from build123d import *

# Parameters (mm, degrees)
BOSS_EXTRUDE1_DEPTH     = 172
BOSS_EXTRUDE2_DEPTH     = 20
SKETCH2_W               = 10
SKETCH2_H               = 13
BOSS_EXTRUDE3_DEPTH     = 15
SKETCH6_W               = 7
SKETCH6_H               = 82.975623271
BOSS_EXTRUDE4_DEPTH     = 15
SKETCH9_W               = 249.172322426
SKETCH9_H               = 172
BOSS_EXTRUDE7_DEPTH     = 20
CUT_EXTRUDE3_DEPTH      = 75
CUT_EXTRUDE3_DEPTH_BACK = 75
SKETCH11_W              = 220
SKETCH11_H              = 130
CUT_EXTRUDE4_DEPTH      = 135
CUT_EXTRUDE4_DEPTH_BACK = 5
SKETCH12_W              = 220
SKETCH12_H              = 10
FILLET2_R               = 70


with BuildPart() as part:
    # Sketch1 → Boss-Extrude1 (new body)
    with BuildSketch(Plane(origin=(0, 0, 0), x_dir=(1, 0, 0), z_dir=(0, 1, 0))):
        Polygon((-125, -75), (-125, -85), (125, -85), (125, 85), (-125, 85), (-125, 75), (115, 75), (115, -75), align=None)
    extrude(amount=BOSS_EXTRUDE1_DEPTH)

    # Sketch1<3> → Boss-Extrude2 (add)
    with BuildSketch(Plane(origin=(0, 0, 0), x_dir=(1, 0, 0), z_dir=(0, 1, 0))):
        Polygon((-195, -85), (-125, -85), (-125, -75), (115, -75), (115, 75), (-125, 75), (-125, 105), (-195, 105), align=None)
    extrude(amount=BOSS_EXTRUDE2_DEPTH)

    # Sketch2 → Boss-Extrude3 (add)
    with BuildSketch(Plane.XY.offset(-75)):
        with Locations((-120, 155.5)):
            Rectangle(SKETCH2_W, SKETCH2_H)
    boss_extrude3 = extrude(amount=BOSS_EXTRUDE3_DEPTH)

    # Sketch5 → CBORE for M3 Hex Head Cap Screw1 (revolve, cut)
    with BuildSketch(Plane(origin=(-115, 156.612141417, -67), x_dir=(0, 0, -1), z_dir=(0, 1, 0))):
        Polygon((0, 0), (0, 80), (1.7, 80), (1.7, 2), (4.6755, 2), (4.6755, 0.025), (4.7005, 0), align=None)
    cbore_for_m3_hex_head_cap_screw1 = revolve(axis=Axis((-108.65, 156.612141417, -67), (-1, 0, 0)), mode=Mode.SUBTRACT)

    # Mirror1: Boss-Extrude3, CBORE for M3 Hex Head Cap Screw1 across plane
    add(boss_extrude3.mirror(Plane.XY))
    add(cbore_for_m3_hex_head_cap_screw1.mirror(Plane.XY), mode=Mode.SUBTRACT)

    # Sketch6 → Boss-Extrude4 (add)
    with BuildSketch(Plane(origin=(0, 0, 75), x_dir=(-1, 0, 0), z_dir=(0, 0, -1))):
        with Locations((110.877553526, 61.319998757)):
            Rectangle(SKETCH6_W, SKETCH6_H)
        with Locations((63.877553526, 61.191761533)):
            Rectangle(SKETCH6_W, SKETCH6_H)
    extrude(amount=BOSS_EXTRUDE4_DEPTH)

    # Sketch9 → Boss-Extrude7 (add)
    with BuildSketch(Plane(origin=(0, 0, -85), x_dir=(-1, 0, 0), z_dir=(0, 0, -1))):
        with Locations((-0.413838787, 86)):
            Rectangle(SKETCH9_W, SKETCH9_H)
    extrude(amount=BOSS_EXTRUDE7_DEPTH)

    # Sketch11 → Cut-Extrude3 (cut, two sides: drawn at the far end of the back side and taken through both)
    with BuildSketch(Plane(origin=(0, 0, -105), x_dir=(-1, 0, 0), z_dir=(0, 0, -1)).offset(-CUT_EXTRUDE3_DEPTH_BACK)):
        with Locations((-0.413838787, 86.484091926)):
            Rectangle(SKETCH11_W, SKETCH11_H)
    extrude(amount=CUT_EXTRUDE3_DEPTH + CUT_EXTRUDE3_DEPTH_BACK, mode=Mode.SUBTRACT)

    # Sketch12 → Cut-Extrude4 (cut, two sides: drawn at the far end of the back side and taken through both)
    with BuildSketch(Plane(origin=(0, 21.484091926, 0), x_dir=(1, 0, 0), z_dir=(0, 1, 0)).offset(-CUT_EXTRUDE4_DEPTH_BACK)):
        with Locations((0.863655378, 99.416077233)):
            Rectangle(SKETCH12_W, SKETCH12_H)
        with Locations((0.307194527, 80.981434553)):
            Rectangle(SKETCH12_W, SKETCH12_H)
    extrude(amount=CUT_EXTRUDE4_DEPTH + CUT_EXTRUDE4_DEPTH_BACK, mode=Mode.SUBTRACT)

    # Fillet2
    fillet2_edges = [part.edges().sort_by_distance(p)[0] for p in [
        (-195, 10, 85),
        (-195, 10, -105),
    ]]
    fillet(fillet2_edges, radius=FILLET2_R - 0.0001)  # a hair under: the kernel refuses the full size


solid = part.part
The listing builds one solid part. Answer for the finished solid, in the listing's coordinates (mm). A direction names the side the tool comes from. Coordinates: 2 decimals unless noted, no trailing zeros. Loops run counter-clockwise (first coordinate to the right, second up) from the corner with the lowest first, then second, coordinate; pieces in that order, holes last.
1) Find the intervals of material crossed by L1, parallel to Y at x = -121.25, z = -67; L2, parallel to Z at x = 24, y = 17.5; L3, parallel to X at y = 132, z = -96, in increasing order.
2) A tool of negligible diameter and unlimited length cuts with its end or side. For faces 1 (the face through (-115, 151, 68)), 2 (the face through (-1, 16.484, -99)), 3 (the face through (110.414, 86, -85)), from which of +Z, -Z, +X, -X, +Y, -Y can it reach the whole face along a straight path? Write none if from no direction.
3) Flat-ended cylindrical pins translate along their axes: pin 1 Ø6 at (y, z) = (92.5, -34) entering from -X; pin 2 Ø8 at (y, z) = (63.5, -75.5) entering from -X; pin 3 Ø4 at (x, y) = (-1, 111.5) entering from -Z. Find the tip coordinate at first contact, or state that the pin passes through.
4) Find section C-C on z = 35.5. Write down the section's boundary in (x, y).
5) Determine the mould class of faces 4 (the face through (-114.378, 61, 68)), 5 (the face through (-117, 157, -65)), 6 (the face through (-33, 0, -9)) for opening direction Y: pulls with the +Y half, pulls with the -Y half, needs draft (parallel to the pull), parting line crosses it, or undercut.
6) Find section B-B on y = 128. Write down the section's boundary in (x, z).
Values:
1. L1: y = 0 to 20, 149 to 154.91, 158.31 to 162
1. L2: z = -105 to -104.42, -94.42 to -85.98, -75.98 to 85
1. L3: x = -124.17 to -109.59, 110.86 to 125
2. face 1: +Y
2. face 2: none
2. face 3: -Z
3. pin 1: stops at x = 115
3. pin 2: stops at x = -125
3. pin 3: stops at z = 75
4. outline: (-191.93, 0) - (125, 0) - (125, 172) - (115, 172) - (115, 20) - (-191.93, 20) - close
5. face 4: needs draft
5. face 5: undercut
5. face 6: pulls with the -Y half
6. outline: (-125, -85) - (-124.17, -85) - (-124.17, -105) - (-109.59, -105) - (-109.59, -85.98) - (-109.69, -85.98) - (-109.69, -75.98) - (-109.59, -75.98) - (-109.59, -75) - (-125, -75) - close; (-125, 75) - (115, 75) - (115, -75) - (110.41, -75) - (110.41, -94.42) - (110.86, -94.42) - (110.86, -104.42) - (110.41, -104.42) - (110.41, -105) - (125, -105) - (125, 85) - (-125, 85) - close
